```python
from build123d import *

# Parameters (mm, degrees)
F0_W     = 200
F0_H     = 150
F1_DEPTH = 17
F2_W     = 200
F2_H     = 10
F3_DEPTH = 12
F2_R     = 4
F2_W_2   = 57.217171
F2_H_2   = 95
F2_W_3   = 112.782829
F2_H_3   = 113
F4_DEPTH = 7
F5_R     = 4
F6_R     = 4
F7_R     = 4


with BuildPart() as f1:
    # F0 (on Top) → F1 (new body)
    with BuildSketch(Plane.XY):
        with Locations((100, 75)):
            Rectangle(F0_W, F0_H)
    extrude(amount=F1_DEPTH)

    # F2 (on face) → F3 (cut)
    with BuildSketch(Plane.XY.offset(17)):
        with Locations((100, 138)):
            Rectangle(F2_W, F2_H)
    extrude(amount=-F3_DEPTH, mode=Mode.SUBTRACT)

    # F2 (on face) → F4 (cut)
    with BuildSketch(Plane.XY.offset(17)):
        with Locations((14, 119)):
            Circle(F2_R)
        with Locations((32, 119)):
            Circle(F2_R)
        with Locations((50, 119)):
            Circle(F2_R)
        with Locations((68, 119)):
            Circle(F2_R)
        with Locations((38.608585, 57.5)):
            Rectangle(F2_W_2, F2_H_2)
        with Locations((133.608586, 66.5)):
            Rectangle(F2_W_3, F2_H_3)
    extrude(amount=-F4_DEPTH, mode=Mode.SUBTRACT)

    # F5
    f5_edges = [f1.edges().sort_by_distance(p)[0] for p in [
        (133.608586, 123, 10),
        (77.217171, 66.5, 10),
        (133.608586, 10, 10),
        (190, 66.5, 10),
    ]]
    fillet(f5_edges, radius=F5_R)

    # F6
    f6_edges = [f1.edges().sort_by_distance(p)[0] for p in [
        (100, 143, 5),
        (100, 133, 5),
    ]]
    fillet(f6_edges, radius=F6_R)

    # F7
    f7_edges = [f1.edges().sort_by_distance(p)[0] for p in [
        (10, 57.5, 10),
        (38.608586, 105, 10),
        (67.217171, 57.5, 10),
        (38.608586, 10, 10),
    ]]
    fillet(f7_edges, radius=F7_R)


solid = f1.part
```
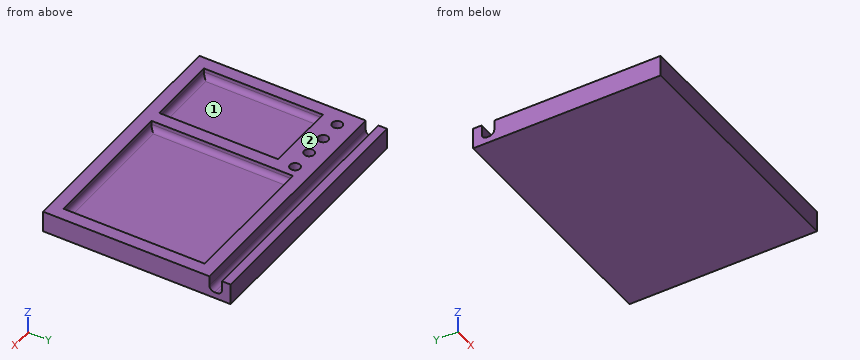
Verification items for the finished model (mm, model axes). Face numbers are marked on the shaded views. A direction names the side the tool comes from. Coordinates: 2 decimals unless noted, no trailing zeros. Loops run counter-clockwise (first coordinate to the right, second up) from the corner with the lowest first, then second, coordinate; pieces in that order, holes last. Notation, with made-up numbers: (11.5, 48) -> (55.5, 48) arc R12 ccw to (55.5, 64) -> close; hole circle Ø2 at (-28, 46). An arc over 180 degrees is marked (long way). Put each result on its own line as item: value.
1. Tool access check on the marked faces 1 and 2. Record the directions out of +Z, -Z, +X, -X, +Y, -Y that give a thin tool (end or side, any length) a straight path to the whole face; none if there is none.
Result set:
face 1: +Z
face 2: +Z, +X, -X, +Y, -Y
2. Section check A-A, the plane x = 149.5. Record the boundary of the cut face in (y, z).
Result set:
outline: (0, 0) -> (150, 0) -> (150, 17) -> (143, 17) -> (143, 9) arc R4 cw to (139, 5) -> (137, 5) arc R4 cw to (133, 9) -> (133, 17) -> (123, 17) -> (123, 14) arc R4 cw to (119, 10) -> (14, 10) arc R4 cw to (10, 14) -> (10, 17) -> (0, 17) -> close
3. Section check C-C, the plane x = 32. Record the boundary of the cut face in (y, z), then the cut area to 3 significant figures.
Result set:
outline: (0, 0) -> (150, 0) -> (150, 17) -> (143, 17) -> (143, 9) arc R4 cw to (139, 5) -> (137, 5) arc R4 cw to (133, 9) -> (133, 17) -> (123, 17) -> (123, 10) -> (115, 10) -> (115, 17) -> (105, 17) -> (105, 14) arc R4 cw to (101, 10) -> (14, 10) arc R4 cw to (10, 14) -> (10, 17) -> (0, 17) -> close
area: 1,720 mm^2
4. Section check B-B, the plane y = 18. Record the boundary of the cut face in (x, z).
Result set:
outline: (0, 0) -> (200, 0) -> (200, 17) -> (190, 17) -> (190, 14) arc R4 cw to (186, 10) -> (81.22, 10) arc R4 cw to (77.22, 14) -> (77.22, 17) -> (67.22, 17) -> (67.22, 14) arc R4 cw to (63.22, 10) -> (14, 10) arc R4 cw to (10, 14) -> (10, 17) -> (0, 17) -> close
5. Thickness scan on line 1 (Y direction, x = 14, z = 14.25); line 2 (Y direction, x = 27, z = 16); line 3 (Y direction, x = 125.5, z = 14). Record the ranges inside material, lowest first.
Result set:
line 1: y = 0 to 10, 105 to 115, 123 to 133, 143 to 150
line 2: y = 0 to 10, 105 to 133, 143 to 150
line 3: y = 0 to 10, 123 to 133, 143 to 150
6. Gauge pin test, flat end, axial feed: P1, Ø4, axis at x = 69, y = 119, coming from the +Z side. Record the tip position at first contact, or that the pin passes through.
Result set:
P1: stops at z = 10
